Verification items for this drawing (mm, ordinates from the low corner). A direction names the side the tool comes from. Give positions to 0.01 mm unless a question says otherwise; leave off trailing zeros. Loops run counter-clockwise (first coordinate to the right, second up) from the corner with the lowest first, then second, coordinate; pieces in that order, holes last. Notation, with made-up numbers: M -38,33 L 20,33 A35 cw 20,65 Z; hole C 24.25,34 d1. An arc over 180 degrees is marked long. Use one line per item in the form item = value.
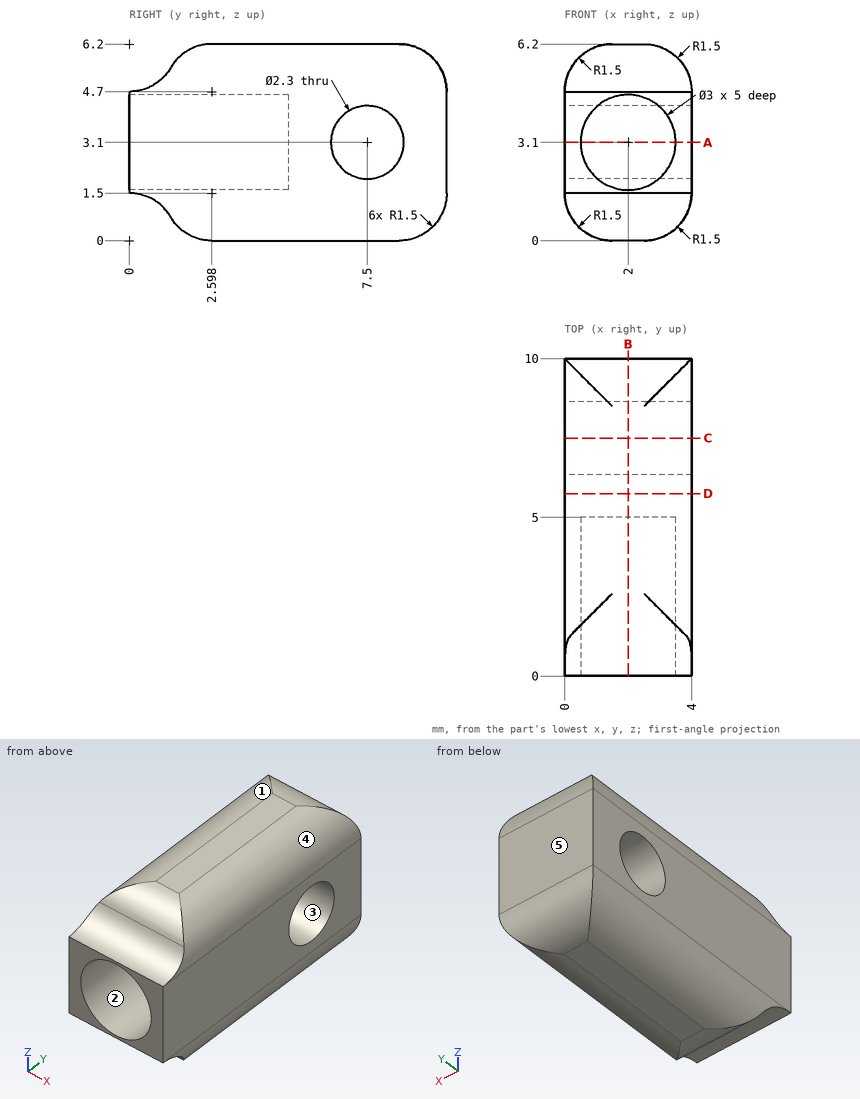
1) Depth check by flat-ended pin: pin 1 Ø1 at (x, y) = (2, 1) entering from +Z. Enter the tip coordinate at first touch or a pass-through.
Evaluation:
pin_1 = 5.72
2) Release check for a two-part mould opening along Y. For the marked faces 3, 4 and 5 record: pulls with the +Y half, pulls with the -Y half, needs draft (parallel to the pull), parting line crosses it, or undercut.
Evaluation:
face_3 = undercut
face_4 = needs draft
face_5 = pulls with the +Y half
3) Section check D-D (y = 5.75). Record the cut outline in (x, z), then the cut area to 3 significant figures.
Evaluation:
outline = M 0,1.5 A1.5 ccw 1.5,0 L 2.5,0 A1.5 ccw 4,1.5 L 4,4.7 A1.5 ccw 2.5,6.2 L 1.5,6.2 A1.5 ccw 0,4.7 Z
area = 22.9 mm^2
4) Section check C-C (y = 7.5). Record the cut outline in (x, z), then the cut area to 3 significant figures.
Evaluation:
outline = M 0,1.5 A1.5 ccw 1.5,0 L 2.5,0 A1.5 ccw 4,1.5 L 4,1.95 L 0,1.95 Z; M 0,4.25 L 4,4.25 L 4,4.7 A1.5 ccw 2.5,6.2 L 1.5,6.2 A1.5 ccw 0,4.7 Z
area = 13.7 mm^2
5) Scan lines: line 1 (Z direction, x = 2, y = 3.1); line 2 (Y direction, x = 3.3, z = 3.5); line 3 (X direction, y = 3, z = 4). Record each from-to range of solid material in increasing order.
Evaluation:
line_1 = 0 to 1.6, 4.6 to 6.2
line_2 = 5 to 6.42, 8.58 to 10
line_3 = 0 to 0.8, 3.2 to 4
6) Section check B-B (x = 2). Record the cut outline in (y, z), then the cut area to 3 significant figures.
Evaluation:
outline = M 0,1.5 A1.5 cw 1.3,0.75 A1.5 ccw 2.6,0 L 8.5,0 A1.5 ccw 10,1.5 L 10,4.7 A1.5 ccw 8.5,6.2 L 2.6,6.2 A1.5 ccw 1.3,5.45 A1.5 cw 0,4.7 L 0,4.6 L 5,4.6 L 5,1.6 L 0,1.6 Z; hole C 7.5,3.1 d2.3
area = 38.0 mm^2
7) Section check A-A (z = 3.1). Record the cut outline in (x, y), then the cut area to 3 significant figures.
Evaluation:
outline = M 0,0 L 0.5,0 L 0.5,5 L 3.5,5 L 3.5,0 L 4,0 L 4,6.35 L 0,6.35 Z; M 0,8.65 L 4,8.65 L 4,10 L 0,10 Z
area = 15.8 mm^2
8) Set-up check for the marked faces 1 and 2: record each of +Z, -Z, +X, -X, +Y, -Y from which the full face is reachable in a straight line by a thin tool's end or side.
Evaluation:
face_1 = +Z, -X, +Y, -Y
face_2 = -Y
